Geometry check sheet. Reference: the model listing, model coordinates, mm. Face numbers are marked on the shaded views. Coordinates: 2 decimals unless noted, no trailing zeros. Order: outer loops, then holes, each group sorted by start corner. A loop starts at its lowest first (then second) coordinate and runs counter-clockwise, first axis right, second up. Notation, with made-up numbers: (75.5, 89) - (92.5, 89) arc R25 ccw to (92.5, 123) - close; hole circle Ø6 at (50, 49). An arc over 180 degrees is marked (long way). Return JSON: item names as keys, results as strings. Group by question number.
Item 1: Section check D-D on z = -95.5. Enter the section's corners in (x, y).
Item 2: Section check C-C on y = 24. Enter the section's corners in (x, z), then the cut area to 3 significant figures.
Item 3: Section check A-A on z = -34. Enter the section's corners in (x, y).
Item 4: Draft check along Z on the marked faces 1 and 2. Enter one of: pulls with the +Z half, pulls with the -Z half, needs draft (parallel to the pull), parting line crosses it, or undercut.
Item 5: Gauge pin test, flat ends, axial feed: pin 1 (13 mm diameter, centred on x = 196.5, y = 17, fed in from +Z); pin 2 (5 mm diameter, centred on x = 158.5, y = 36, fed in from -Z); pin 3 (13 mm diameter, centred on x = 7.5, y = 16, fed in from -Z). Record the tip position at first contact, or that the pin passes through.
Item 6: Section check B-B on x = 95. Enter the section's corners in (y, z).
Item 7: Scan lines: probe 1 along X at (y, z) = (8, 57.5); probe 2 along Z at (x, y) = (35.5, 36.5); probe 3 along Z at (x, y) = (158.5, 19.5). Record each from-to range of solid material in increasing order.
Autodesk Inventor part; units mm, degrees
ref_plane "YZ Plane" through (0, 0, 0) normal (1, 0, 0) x (0, 1, 0)
ref_plane "XZ Plane" through (0, 0, 0) normal (0, 1, 0) x (-1, 0, 0)
ref_plane "XY Plane" through (0, 0, 0) normal (0, 0, 1) x (1, 0, 0)
sketch "Эскиз1" plane through (0, 0, 0) normal (1, 0, 0) x (0, 1, 0)
  line L0 (29, 218.9091) -> (0, 218.9091)
  line L1 (0, 218.9091) -> (0, -297.0909)
  line L2 (0, -297.0909) -> (29, -297.0909)
  line L3 (29, -297.0909) -> (29, 218.9091)
  point P0 (0, 0)
  dimension "d0" = 516
  dimension "d1" = 29
extrude "Выдавливание1" add sketch "Эскиз1" along normal blind 200
sketch "Эскиз2" plane through (0, 29, 218.9091) normal (0, 1, 0) x (1, 0, 0)
  line L0 (0, 516) -> (0, 0)
  line L1 (0, 0) -> (200, 0)
  line L2 (200, 516) -> (200, 0)
  line L3 (0, 516) -> (200, 516)
  line L4 (20, 232) -> (180, 232)
  line L5 (180, 232) -> (180, 284)
  line L6 (180, 284) -> (20, 284)
  line L7 (20, 284) -> (20, 232)
  line L8 (20, 232) -> (180, 232)
  line L9 (180, 232) -> (180, 222)
  line L10 (180, 222) -> (20, 222)
  line L11 (20, 222) -> (20, 232)
  line L12 (20, 284) -> (180, 284)
  line L13 (180, 284) -> (180, 294)
  line L14 (180, 294) -> (20, 294)
  line L15 (20, 294) -> (20, 284)
  line L16 (70, 232) -> (130, 232)
  line L17 (130, 232) -> (130, 284)
  line L18 (130, 284) -> (70, 284)
  line L19 (70, 284) -> (70, 232)
  circle A0 centre (70, 236) radius 4
  circle A1 centre (70, 280) radius 4
  circle A2 centre (130, 280) radius 4
  circle A3 centre (130, 236) radius 4
  point P0 (0, 218.9091)
  point P1 (130, 240)
  point P2 (130, 276)
  point P3 (70, 276)
  point P4 (70, 240)
  dimension "d4" = 52
  dimension "d5" = 20
  dimension "d6" = 20
  dimension "d7" = 232
  dimension "d8" = 232
  dimension "d9" = 10
  dimension "d10" = 10
  dimension "d11" = 50
  dimension "d12" = 50
extrude "Выдавливание2" add sketch "Эскиз2" along normal blind 10 contours L4 L9 L10 L11 | A0 L19 A1 L6 A2 L17 A3 L4 | L15 L14 L13 L6
sketch "Эскиз3" plane through (0, 29, 218.9091) normal (0, 1, 0) x (1, 0, 0)
  line L0 (180, 294) -> (180, 284)
  line L1 (180, 284) -> (130, 284)
  arc A0 (130, 284) -> (130, 276) centre (130, 280) ccw
  line L2 (130, 276) -> (130, 240)
  arc A1 (130, 240) -> (130, 232) centre (130, 236) ccw
  line L3 (130, 232) -> (180, 232)
  line L4 (180, 232) -> (180, 222)
  line L5 (180, 222) -> (20, 222)
  line L6 (20, 222) -> (20, 232)
  line L7 (20, 232) -> (70, 232)
  arc A2 (70, 232) -> (70, 240) centre (70, 236) ccw
  line L8 (70, 240) -> (70, 276)
  arc A3 (70, 276) -> (70, 284) centre (70, 280) ccw
  line L9 (70, 284) -> (20, 284)
  line L10 (20, 284) -> (20, 294)
  line L11 (20, 294) -> (180, 294)
  line L12 (0, 516) -> (0, 0)
  line L13 (0, 0) -> (200, 0)
  line L14 (200, 516) -> (200, 0)
  line L15 (0, 516) -> (200, 516)
  line L16 (12, 12) -> (12, 504)
  line L17 (12, 504) -> (188, 504)
  line L18 (188, 504) -> (188, 12)
  line L19 (188, 12) -> (12, 12)
  line L20 (8, 210) -> (192, 210)
  line L21 (192, 210) -> (192, 244)
  line L22 (192, 244) -> (142, 244)
  line L23 (142, 244) -> (142, 272)
  line L24 (142, 272) -> (192, 272)
  line L25 (192, 272) -> (192, 306)
  line L26 (192, 306) -> (8, 306)
  line L27 (8, 306) -> (8, 272)
  line L28 (8, 272) -> (58, 272)
  line L29 (58, 272) -> (58, 244)
  line L30 (58, 244) -> (8, 244)
  line L31 (8, 244) -> (8, 210)
  line L32 (-28, 416) -> (286, 416)
  line L33 (286, 416) -> (286, 100)
  line L34 (286, 100) -> (-28, 100)
  line L35 (-28, 100) -> (-28, 416)
  point P0 (0, 218.9091)
  point P1 (0, 416)
  point P2 (12, 416)
  point P3 (12, 306)
  point P4 (188, 306)
  point P5 (188, 416)
  point P6 (200, 416)
  point P7 (200, 100)
  point P8 (188, 100)
  point P9 (188, 210)
  point P10 (12, 210)
  point P11 (12, 100)
  point P12 (0, 100)
  dimension "d15" = 100
  dimension "d16" = 100
extrude "Выдавливание3" cut sketch "Эскиз3" against normal blind 25 contours L15 L14 L32 L18 L17 L16 L12 | L34 L16 L19 L18 L14 L13 L12 | L32 L18 L26 L16 | L16 L17 L18 L32 | L34 L18 L19 L16 | L16 L20 L18 L34
sketch "Эскиз4" plane through (200, 0, 0) normal (1, 0, 0) x (0, 0, -1)
  line L0 (-218.9091, 0) -> (-215.9091, 0)
  line L1 (-215.9091, 0) -> (-215.9091, 13.6393)
  line L2 (-215.9091, 13.6393) -> (-218.9091, 13.6393)
  line L3 (-218.9091, 13.6393) -> (-218.9091, 0)
  line L4 (297.0909, 0) -> (297.0909, 4)
  line L5 (297.0909, 0) -> (294.0909, 0)
  line L6 (294.0909, 0) -> (294.0909, 8)
  line L7 (294.0909, 8) -> (297.0909, 8)
  line L8 (297.0909, 8) -> (297.0909, 0)
  point P0 (0, 0)
  dimension "d19" = 3
  dimension "d20" = 3
extrude "Выдавливание4" cut sketch "Эскиз4" against normal blind 1000
properties part number "Niz_Plita" material "Алюминий 6061"
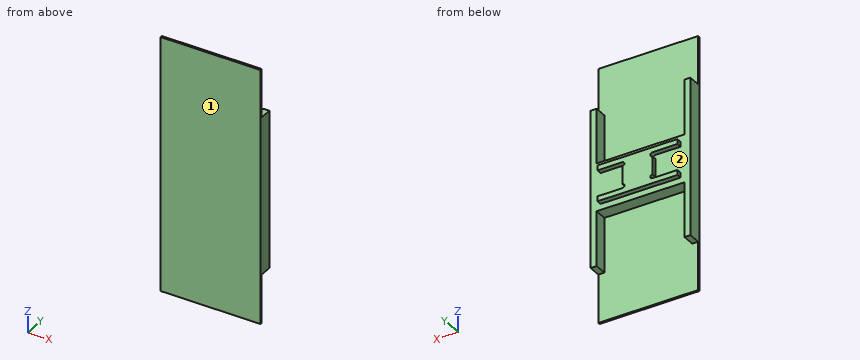
Computed:
{
 "1": {"outline": "(0, 0) - (200, 0) - (200, 29) - (188, 29) - (188, 4) - (12, 4) - (12, 29) - (0, 29) - close"},
 "2": {"outline": "(0, -197.09) - (12, -197.09) - (12, -87.09) - (188, -87.09) - (188, -197.09) - (200, -197.09) - (200, 118.91) - (188, 118.91) - (188, 8.91) - (12, 8.91) - (12, 118.91) - (0, 118.91) - close", "area": "24,500 mm²"},
 "3": {"outline": "(0, 0) - (200, 0) - (200, 29) - (130, 29) - (130, 39) - (70, 39) - (70, 29) - (0, 29) - close"},
 "4": {"face 1": "needs draft", "face 2": "undercut"},
 "5": {"pin 1": "stops at z = 118.91", "pin 2": "stops at z = -75.09", "pin 3": "stops at z = -197.09"},
 "6": {"outline": "(0, -294.09) - (4, -294.09) - (4, -87.09) - (29, -87.09) - (29, -75.09) - (39, -75.09) - (39, -3.09) - (29, -3.09) - (29, 8.91) - (4, 8.91) - (4, 215.91) - (0, 215.91) - close"},
 "7": {"probe 1": "x = 0 to 12, 188 to 200", "probe 2": "z = -75.09 to -65.09, -13.09 to -3.09", "probe 3": "z = -87.09 to 8.91"}
}
